Check sheet for the drawn part. Datum: minimum x, y, z corner. Units: mm. A direction names the side the tool comes from. Coordinates: 2 decimals unless noted, no trailing zeros. Loops run counter-clockwise (first coordinate to the right, second up) from the corner with the lowest first, then second, coordinate; pieces in that order, holes last. Notation, with made-up numbers: M 25.25,-30.75 L 57.25,-30.75 A22 ccw 57.25,-9.75 Z; hole C -4.5,20 d2. An arc over 180 degrees is marked long. Use CSV: the item, a comma, the result in double quotes. Start each with the question number.
(1) Section check B-B on z = 15. Record the cut outline in (x, y).
(2) Section check C-C on y = 116. Record the cut outline in (x, z).
(3) Go/stop test with flat-tipped pins: pin 1 Ø1.5 at (x, y) = (18, 47.5) entering from +Z; pin 2 Ø8 at (y, z) = (155, 18.5) entering from -X; pin 3 Ø9 at (x, z) = (81, 18) entering from -Y. Record where each tip stops, or that it passes through.
(4) Section check A-A on x = 67.5. Record the cut outline in (y, z), and give its area (3 significant figures).
(5) Set-up check for the marked faces 1 and 2: record each of +Z, -Z, +X, -X, +Y, -Y from which the full face is reachable in a straight line by a thin tool's end or side.
(6) Section check D-D on x = 15.5. Record the cut outline in (y, z).
(7) Scan lines: line 1 (X direction, y = 158, z = 15); line 2 (Z direction, x = 67, y = 157); line 3 (Y direction, x = 85, z = 11). Record each from-to range of solid material in increasing order.
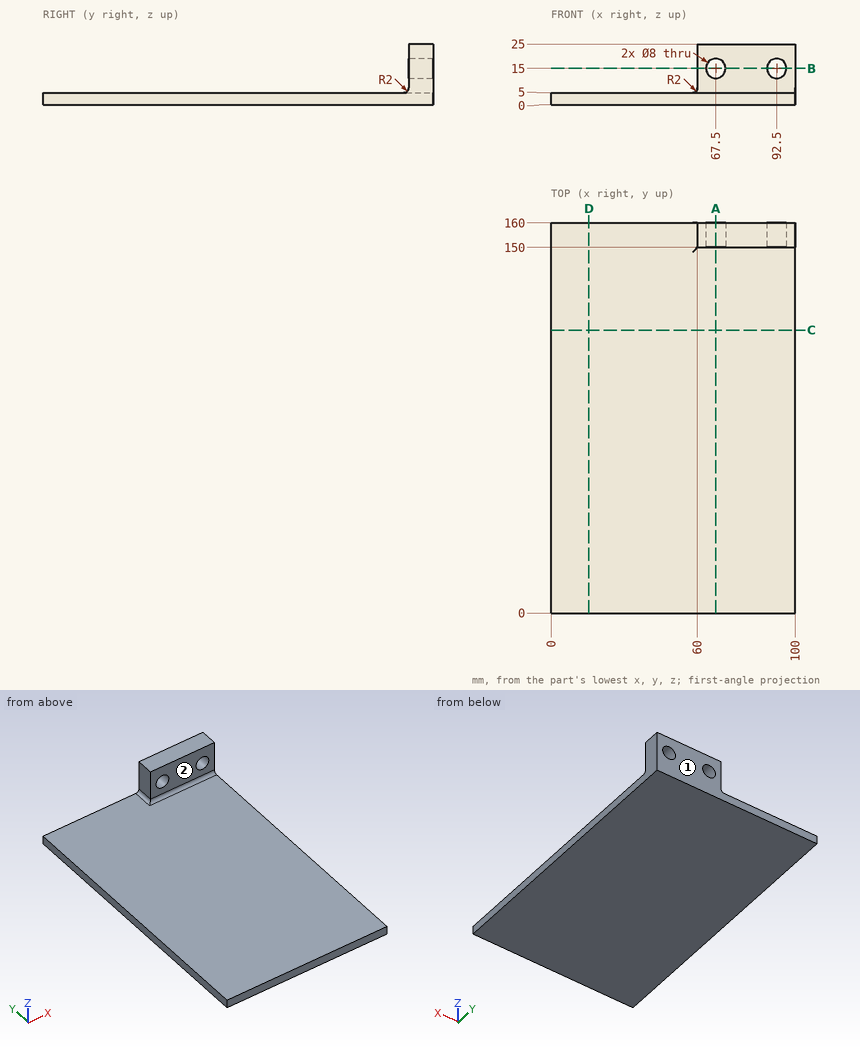
Outcome:
1,outline,"M 60,150 L 63.5,150 L 63.5,160 L 60,160 Z; M 71.5,150 L 88.5,150 L 88.5,160 L 71.5,160 Z; M 96.5,150 L 100,150 L 100,160 L 96.5,160 Z"
2,outline,"M 0,0 L 100,0 L 100,5 L 0,5 Z"
3,pin 1,"stops at z = 5"
3,pin 2,"stops at x = 60"
3,pin 3,"stops at y = 150"
4,outline,"M 0,0 L 160,0 L 160,11 L 150,11 L 150,7 A2 cw 148,5 L 0,5 Z; M 150,19 L 160,19 L 160,25 L 150,25 Z"
4,area,"921 mm²"
5,face 1,"+Z, -Z, +X, -X, +Y"
5,face 2,"+Z, +X, -X, -Y"
6,outline,"M 0,0 L 160,0 L 160,5 L 0,5 Z"
7,line 1,"x = 60 to 63.5, 71.5 to 88.5, 96.5 to 100"
7,line 2,"z = 0 to 11.03, 18.97 to 25"
7,line 3,"y = 150 to 160"
